Design review of the part built by this model. Coordinates are the model's own, in mm. A direction names the side the tool comes from. Give positions to 0.01 mm unless a question says otherwise; leave off trailing zeros. Loops run counter-clockwise (first coordinate to the right, second up) from the corner with the lowest first, then second, coordinate; pieces in that order, holes last.
from build123d import *

# Parameters (mm, degrees)
SKETCH2_R   = 6
SKETCH2_R_2 = 4.5


with BuildPart() as part:
    # Sweep1: sweep along a curve in space
    with BuildLine() as sweep1_path:
        Line((0, 0, 0), (0, -60.373066959, 0))
        ThreePointArc((0, -60.373066959, 0), (0.715557648, -65.808266906, 0), (2.813466521, -70.873066959, 0))
        Line((2.813466521, -70.873066959, 0), (27.186533479, -113.088457268, 0))
        ThreePointArc((27.186533479, -113.088457268, 0), (29.284442352, -118.153257321, 0), (30, -123.588457268, 0))
        Line((30, -123.588457268, 0), (30, -672.73491671, 0))
        ThreePointArc((30, -672.73491671, 0), (30, -679.91733972, 1.266454963), (30, -686.233456513, 4.913066695))
        Line((30, -686.233456513, 4.913066695), (30, -739.344889262, 49.478850325))
        ThreePointArc((30, -739.344889262, 49.478850325), (32.668913393, -746.748845442, 58.094607638), (39.851540684, -749.5, 66.870367075))
        Line((39.851540684, -749.5, 66.870367075), (86.085931999, -749.5, 108.5))
    # Sketch2 → Sweep1 (sweep)
    with BuildSketch(Plane(origin=(0, 0, 0), x_dir=(1, 0, 0), z_dir=(0, 1, 0))):
        Circle(SKETCH2_R)
        Circle(SKETCH2_R_2, mode=Mode.SUBTRACT)
    sweep(path=sweep1_path.line)


solid = part.part
Q1. Insertion check: pin 1 (1.5 mm diameter, centred on x = 31, z = 18.5, fed in from +Y); pin 2 (1 mm diameter, centred on y = -315, z = 6, fed in from +X); pin 3 (10.5 mm diameter, centred on x = 30, z = 0, fed in from -Y). Each pin has a flat end and moves straight along its axis. Give the tip position at first contact, or say it passes through.
Results:
pin 1: stops at y = -692.31
pin 2: stops at x = 32.4
pin 3: stops at y = -695.97
Q2. Wall thickness on line 1 (Z direction, x = 0, y = -32); line 2 (X direction, y = -329, z = 0); line 3 (X direction, y = -59.5, z = 4): over which ranges is each line inside the solid? List them lowest first.
Results:
line 1: z = -6 to -4.5, 4.5 to 6
line 2: x = 24 to 25.5, 34.5 to 36
line 3: x = -4.47 to -2.06, 2.06 to 4.47
Q3. Tool access review of faces 5 (the face through (24, -402, 0)), 6 (the face through (-6, -31, 0)): name each direction out of +Z, -Z, +X, -X, +Y, -Y from which nothing blocks a thin tool from reaching the whole face with its end or side.
Results:
face 5: none
face 6: +Y
Q4. Take a section at A-A (y = -576.5). Give the boundary of the cut face in (x, z), plus the area to 3 significant figures.
Results:
outline: circle Ø12 at (30, 0); hole circle Ø9 at (30, 0)
area: 49.5 mm2
Q5. Draft analysis for pull direction X (two halves, no side actions). For faces 1 (the face through (28.7, -716.9, 23)), 2 (the face through (63.767, -745.056, 87.45)), 3 (the face through (4.5, 0, -1.4)), 4 (the face through (11.277, -94.524, 0.198)), state which applies: pulls with the +X half, pulls with the -X half, needs draft (parallel to the pull), parting line crosses it, or undercut.
Results:
face 1: parting line crosses it
face 2: undercut
face 3: needs draft
face 4: undercut
